```python
from build123d import *

# Parameters (mm, degrees)
BOSS_EXTRUDE1_DEPTH = 80
CUT_EXTRUDE1_REACH  = 152.333
CUT_EXTRUDE2_REACH  = 152.333
CUT_EXTRUDE3_REACH  = 152.333
SKETCH4_R           = 3
CUT_EXTRUDE4_REACH  = 152.333
SKETCH5_R           = 2.5
SKETCH5_R_2         = 3


with BuildPart() as part:
    # Sketch1 → Boss-Extrude1 (new body)
    with BuildSketch(Plane(origin=(0, 0, 0), x_dir=(1, 0, 0), z_dir=(0, 1, 0))):
        Polygon((0, 0), (90, 0), (90, 10), (10, 10), (10, 90), (0, 90), align=None)
    extrude(amount=BOSS_EXTRUDE1_DEPTH)

    # Sketch2 → Cut-Extrude1 (cut, up to next)
    with BuildSketch(Plane.XY, mode=Mode.PRIVATE) as cut_extrude1_sk1:
        Polygon((45, 80), (90, 40), (90, 80), align=None)
    cut_extrude1_tool1 = extrude(cut_extrude1_sk1.sketch, amount=-CUT_EXTRUDE1_REACH, mode=Mode.PRIVATE) & part.part
    add(cut_extrude1_tool1.solids().sort_by_distance((75, 66.666667, 0))[0], mode=Mode.SUBTRACT)

    # Sketch3 → Cut-Extrude2 (cut, up to next)
    with BuildSketch(Plane.ZY, mode=Mode.PRIVATE) as cut_extrude2_sk1:
        Polygon((-45, 80), (-90, 40), (-90, 80), align=None)
    cut_extrude2_tool1 = extrude(cut_extrude2_sk1.sketch, amount=-CUT_EXTRUDE2_REACH, mode=Mode.PRIVATE) & part.part
    add(cut_extrude2_tool1.solids().sort_by_distance((0, 66.666667, -75))[0], mode=Mode.SUBTRACT)

    # Sketch4 → Cut-Extrude3 (cut, up to next)
    with BuildSketch(Plane.XY, mode=Mode.PRIVATE) as cut_extrude3_sk1:
        with Locations((20, 70)):
            Circle(SKETCH4_R)
    cut_extrude3_tool1 = extrude(cut_extrude3_sk1.sketch, amount=-CUT_EXTRUDE3_REACH, mode=Mode.PRIVATE) & part.part
    # Sketch4 → Cut-Extrude3 (cut, up to next)
    with BuildSketch(Plane.XY, mode=Mode.PRIVATE) as cut_extrude3_sk2:
        with Locations((40, 70)):
            Circle(SKETCH4_R)
    cut_extrude3_tool2 = extrude(cut_extrude3_sk2.sketch, amount=-CUT_EXTRUDE3_REACH, mode=Mode.PRIVATE) & part.part
    # Sketch4 → Cut-Extrude3 (cut, up to next)
    with BuildSketch(Plane.XY, mode=Mode.PRIVATE) as cut_extrude3_sk3:
        with Locations((40, 50)):
            Circle(SKETCH4_R)
    cut_extrude3_tool3 = extrude(cut_extrude3_sk3.sketch, amount=-CUT_EXTRUDE3_REACH, mode=Mode.PRIVATE) & part.part
    # Sketch4 → Cut-Extrude3 (cut, up to next)
    with BuildSketch(Plane.XY, mode=Mode.PRIVATE) as cut_extrude3_sk4:
        with Locations((20, 30)):
            Circle(SKETCH4_R)
    cut_extrude3_tool4 = extrude(cut_extrude3_sk4.sketch, amount=-CUT_EXTRUDE3_REACH, mode=Mode.PRIVATE) & part.part
    # Sketch4 → Cut-Extrude3 (cut, up to next)
    with BuildSketch(Plane.XY, mode=Mode.PRIVATE) as cut_extrude3_sk5:
        with Locations((40, 10)):
            Circle(SKETCH4_R)
    cut_extrude3_tool5 = extrude(cut_extrude3_sk5.sketch, amount=-CUT_EXTRUDE3_REACH, mode=Mode.PRIVATE) & part.part
    # Sketch4 → Cut-Extrude3 (cut, up to next)
    with BuildSketch(Plane.XY, mode=Mode.PRIVATE) as cut_extrude3_sk6:
        with Locations((20, 50)):
            Circle(SKETCH4_R)
    cut_extrude3_tool6 = extrude(cut_extrude3_sk6.sketch, amount=-CUT_EXTRUDE3_REACH, mode=Mode.PRIVATE) & part.part
    # Sketch4 → Cut-Extrude3 (cut, up to next)
    with BuildSketch(Plane.XY, mode=Mode.PRIVATE) as cut_extrude3_sk7:
        with Locations((40, 30)):
            Circle(SKETCH4_R)
    cut_extrude3_tool7 = extrude(cut_extrude3_sk7.sketch, amount=-CUT_EXTRUDE3_REACH, mode=Mode.PRIVATE) & part.part
    # Sketch4 → Cut-Extrude3 (cut, up to next)
    with BuildSketch(Plane.XY, mode=Mode.PRIVATE) as cut_extrude3_sk8:
        with Locations((20, 10)):
            Circle(SKETCH4_R)
    cut_extrude3_tool8 = extrude(cut_extrude3_sk8.sketch, amount=-CUT_EXTRUDE3_REACH, mode=Mode.PRIVATE) & part.part
    # Sketch4 → Cut-Extrude3 (cut, up to next)
    with BuildSketch(Plane.XY, mode=Mode.PRIVATE) as cut_extrude3_sk9:
        with Locations((60, 30)):
            Circle(SKETCH4_R)
    cut_extrude3_tool9 = extrude(cut_extrude3_sk9.sketch, amount=-CUT_EXTRUDE3_REACH, mode=Mode.PRIVATE) & part.part
    # Sketch4 → Cut-Extrude3 (cut, up to next)
    with BuildSketch(Plane.XY, mode=Mode.PRIVATE) as cut_extrude3_sk10:
        with Locations((80, 10)):
            Circle(SKETCH4_R)
    cut_extrude3_tool10 = extrude(cut_extrude3_sk10.sketch, amount=-CUT_EXTRUDE3_REACH, mode=Mode.PRIVATE) & part.part
    # Sketch4 → Cut-Extrude3 (cut, up to next)
    with BuildSketch(Plane.XY, mode=Mode.PRIVATE) as cut_extrude3_sk11:
        with Locations((80, 30)):
            Circle(SKETCH4_R)
    cut_extrude3_tool11 = extrude(cut_extrude3_sk11.sketch, amount=-CUT_EXTRUDE3_REACH, mode=Mode.PRIVATE) & part.part
    # Sketch4 → Cut-Extrude3 (cut, up to next)
    with BuildSketch(Plane.XY, mode=Mode.PRIVATE) as cut_extrude3_sk12:
        with Locations((60, 10)):
            Circle(SKETCH4_R)
    cut_extrude3_tool12 = extrude(cut_extrude3_sk12.sketch, amount=-CUT_EXTRUDE3_REACH, mode=Mode.PRIVATE) & part.part
    add(cut_extrude3_tool1.solids().sort_by_distance((20, 70, 0))[0], mode=Mode.SUBTRACT)
    add(cut_extrude3_tool2.solids().sort_by_distance((40, 70, 0))[0], mode=Mode.SUBTRACT)
    add(cut_extrude3_tool3.solids().sort_by_distance((40, 50, 0))[0], mode=Mode.SUBTRACT)
    add(cut_extrude3_tool4.solids().sort_by_distance((20, 30, 0))[0], mode=Mode.SUBTRACT)
    add(cut_extrude3_tool5.solids().sort_by_distance((40, 10, 0))[0], mode=Mode.SUBTRACT)
    add(cut_extrude3_tool6.solids().sort_by_distance((20, 50, 0))[0], mode=Mode.SUBTRACT)
    add(cut_extrude3_tool7.solids().sort_by_distance((40, 30, 0))[0], mode=Mode.SUBTRACT)
    add(cut_extrude3_tool8.solids().sort_by_distance((20, 10, 0))[0], mode=Mode.SUBTRACT)
    add(cut_extrude3_tool9.solids().sort_by_distance((60, 30, 0))[0], mode=Mode.SUBTRACT)
    add(cut_extrude3_tool10.solids().sort_by_distance((80, 10, 0))[0], mode=Mode.SUBTRACT)
    add(cut_extrude3_tool11.solids().sort_by_distance((80, 30, 0))[0], mode=Mode.SUBTRACT)
    add(cut_extrude3_tool12.solids().sort_by_distance((60, 10, 0))[0], mode=Mode.SUBTRACT)

    # Sketch5 → Cut-Extrude4 (cut, up to next)
    with BuildSketch(Plane.ZY, mode=Mode.PRIVATE) as cut_extrude4_sk1:
        with Locations((-20, 30)):
            Circle(SKETCH5_R)
    cut_extrude4_tool1 = extrude(cut_extrude4_sk1.sketch, amount=-CUT_EXTRUDE4_REACH, mode=Mode.PRIVATE) & part.part
    # Sketch5 → Cut-Extrude4 (cut, up to next)
    with BuildSketch(Plane.ZY, mode=Mode.PRIVATE) as cut_extrude4_sk2:
        with Locations((-40, 30)):
            Circle(SKETCH5_R)
    cut_extrude4_tool2 = extrude(cut_extrude4_sk2.sketch, amount=-CUT_EXTRUDE4_REACH, mode=Mode.PRIVATE) & part.part
    # Sketch5 → Cut-Extrude4 (cut, up to next)
    with BuildSketch(Plane.ZY, mode=Mode.PRIVATE) as cut_extrude4_sk3:
        with Locations((-40, 10)):
            Circle(SKETCH5_R)
    cut_extrude4_tool3 = extrude(cut_extrude4_sk3.sketch, amount=-CUT_EXTRUDE4_REACH, mode=Mode.PRIVATE) & part.part
    # Sketch5 → Cut-Extrude4 (cut, up to next)
    with BuildSketch(Plane.ZY, mode=Mode.PRIVATE) as cut_extrude4_sk4:
        with Locations((-20, 10)):
            Circle(SKETCH5_R)
    cut_extrude4_tool4 = extrude(cut_extrude4_sk4.sketch, amount=-CUT_EXTRUDE4_REACH, mode=Mode.PRIVATE) & part.part
    # Sketch5 → Cut-Extrude4 (cut, up to next)
    with BuildSketch(Plane.ZY, mode=Mode.PRIVATE) as cut_extrude4_sk5:
        with Locations((-20, 70)):
            Circle(SKETCH5_R_2)
    cut_extrude4_tool5 = extrude(cut_extrude4_sk5.sketch, amount=-CUT_EXTRUDE4_REACH, mode=Mode.PRIVATE) & part.part
    # Sketch5 → Cut-Extrude4 (cut, up to next)
    with BuildSketch(Plane.ZY, mode=Mode.PRIVATE) as cut_extrude4_sk6:
        with Locations((-40, 70)):
            Circle(SKETCH5_R_2)
    cut_extrude4_tool6 = extrude(cut_extrude4_sk6.sketch, amount=-CUT_EXTRUDE4_REACH, mode=Mode.PRIVATE) & part.part
    # Sketch5 → Cut-Extrude4 (cut, up to next)
    with BuildSketch(Plane.ZY, mode=Mode.PRIVATE) as cut_extrude4_sk7:
        with Locations((-40, 50)):
            Circle(SKETCH5_R_2)
    cut_extrude4_tool7 = extrude(cut_extrude4_sk7.sketch, amount=-CUT_EXTRUDE4_REACH, mode=Mode.PRIVATE) & part.part
    # Sketch5 → Cut-Extrude4 (cut, up to next)
    with BuildSketch(Plane.ZY, mode=Mode.PRIVATE) as cut_extrude4_sk8:
        with Locations((-20, 50)):
            Circle(SKETCH5_R_2)
    cut_extrude4_tool8 = extrude(cut_extrude4_sk8.sketch, amount=-CUT_EXTRUDE4_REACH, mode=Mode.PRIVATE) & part.part
    # Sketch5 → Cut-Extrude4 (cut, up to next)
    with BuildSketch(Plane.ZY, mode=Mode.PRIVATE) as cut_extrude4_sk9:
        with Locations((-60, 30)):
            Circle(SKETCH5_R_2)
    cut_extrude4_tool9 = extrude(cut_extrude4_sk9.sketch, amount=-CUT_EXTRUDE4_REACH, mode=Mode.PRIVATE) & part.part
    # Sketch5 → Cut-Extrude4 (cut, up to next)
    with BuildSketch(Plane.ZY, mode=Mode.PRIVATE) as cut_extrude4_sk10:
        with Locations((-80, 30)):
            Circle(SKETCH5_R_2)
    cut_extrude4_tool10 = extrude(cut_extrude4_sk10.sketch, amount=-CUT_EXTRUDE4_REACH, mode=Mode.PRIVATE) & part.part
    # Sketch5 → Cut-Extrude4 (cut, up to next)
    with BuildSketch(Plane.ZY, mode=Mode.PRIVATE) as cut_extrude4_sk11:
        with Locations((-80, 10)):
            Circle(SKETCH5_R_2)
    cut_extrude4_tool11 = extrude(cut_extrude4_sk11.sketch, amount=-CUT_EXTRUDE4_REACH, mode=Mode.PRIVATE) & part.part
    # Sketch5 → Cut-Extrude4 (cut, up to next)
    with BuildSketch(Plane.ZY, mode=Mode.PRIVATE) as cut_extrude4_sk12:
        with Locations((-60, 10)):
            Circle(SKETCH5_R_2)
    cut_extrude4_tool12 = extrude(cut_extrude4_sk12.sketch, amount=-CUT_EXTRUDE4_REACH, mode=Mode.PRIVATE) & part.part
    add(cut_extrude4_tool1.solids().sort_by_distance((0, 30, -20))[0], mode=Mode.SUBTRACT)
    add(cut_extrude4_tool2.solids().sort_by_distance((0, 30, -40))[0], mode=Mode.SUBTRACT)
    add(cut_extrude4_tool3.solids().sort_by_distance((0, 10, -40))[0], mode=Mode.SUBTRACT)
    add(cut_extrude4_tool4.solids().sort_by_distance((0, 10, -20))[0], mode=Mode.SUBTRACT)
    add(cut_extrude4_tool5.solids().sort_by_distance((0, 70, -20))[0], mode=Mode.SUBTRACT)
    add(cut_extrude4_tool6.solids().sort_by_distance((0, 70, -40))[0], mode=Mode.SUBTRACT)
    add(cut_extrude4_tool7.solids().sort_by_distance((0, 50, -40))[0], mode=Mode.SUBTRACT)
    add(cut_extrude4_tool8.solids().sort_by_distance((0, 50, -20))[0], mode=Mode.SUBTRACT)
    add(cut_extrude4_tool9.solids().sort_by_distance((0, 30, -60))[0], mode=Mode.SUBTRACT)
    add(cut_extrude4_tool10.solids().sort_by_distance((0, 30, -80))[0], mode=Mode.SUBTRACT)
    add(cut_extrude4_tool11.solids().sort_by_distance((0, 10, -80))[0], mode=Mode.SUBTRACT)
    add(cut_extrude4_tool12.solids().sort_by_distance((0, 10, -60))[0], mode=Mode.SUBTRACT)


solid = part.part
```
Read the model definition and answer for the solid it produces. Units are mm, in the model's axes. A direction names the side the tool comes from. Coordinates: 2 decimals unless noted, no trailing zeros. Order: outer loops, then holes, each group sorted by start corner. A loop starts at its lowest first (then second) coordinate and runs counter-clockwise, first axis right, second up. Notation, with made-up numbers: (-14, 77) - (21, 77) arc R16 cw to (21, 91) - close; hole circle Ø5 at (13, 3). An arc over 180 degrees is marked (long way). Answer as a JSON object with one key per item and string values. Group by question number.
Item 1: Section C-C (x = 60) is taken. Give the vertices of the cut face in (y, z), plus the area to 3 significant figures.
Item 2: Section A-A (y = 70) is taken. Give the vertices of the cut face in (x, z), plus the area to 3 significant figures.
Item 3: Consider probe 1 along Y at (x, z) = (20, -8); probe 2 along Y at (x, z) = (2, -60); probe 3 along Y at (x, z) = (7, -62). Determine where each line is inside the solid, lowest interval first. Write a range as from..to.
Item 4: Flat-ended cylindrical pins translate along their axes: P1, Ø5, axis at y = 23, z = -30, coming from the -X side; P2, Ø24, axis at x = 65.5, y = 36, coming from the -Z side; P3, Ø6.5, axis at y = 10, z = -20, coming from the +X side. Find the tip coordinate at first contact, or state that the pin passes through.
Item 5: Section D-D (z = -60) is taken. Give the vertices of the cut face in (x, y).
Item 6: The mould has two halves that part along Z. Classify faces 1 (the face through (5, 53, -20)), 2 (the face through (57, 30, -5)), 3 (the face through (42, 39, -10)): +Z half, -Z half, draft (parallel to the pull), parting line (faces both ways), or undercut.
Item 7: Section B-B (z = -20) is taken. Give the vertices of the cut face in (x, y), plus the area to 3 significant figures.
Item 8: A tool of negligible diameter and unlimited length cuts with its end or side. For faces 4 (the face through (10, 39, -49)), 5 (the face through (19.35, 67.07, -4.93)), from which of +Z, -Z, +X, -X, +Y, -Y can it reach the whole face along a straight path? Write none if from no direction.
Results are:
{
 "1": {"outline": "(0, -10) - (7, -10) - (7, 0) - (0, 0) - close; (13, -10) - (27, -10) - (27, 0) - (13, 0) - close; (33, -10) - (66.67, -10) - (66.67, 0) - (33, 0) - close", "area": "547 mm^2"},
 "2": {"outline": "(0, -56.25) - (10, -56.25) - (10, -43) - (0, -43) - close; (0, -37) - (10, -37) - (10, -23) - (0, -23) - close; (0, -17) - (10, -17) - (10, -10) - (17, -10) - (17, 0) - (0, 0) - close; (23, -10) - (37, -10) - (37, 0) - (23, 0) - close; (43, -10) - (56.25, -10) - (56.25, 0) - (43, 0) - close", "area": "785 mm^2"},
 "3": {"probe 1": "y = 0..7, 13..27, 33..47, 53..67, 73..80", "probe 2": "y = 0..7, 13..27, 33..66.67", "probe 3": "y = 0..7.76, 12.24..27.76, 32.24..64.89"},
 "4": {"P1": "stops at x = 0", "P2": "stops at z = -10", "P3": "stops at x = 10"},
 "5": {"outline": "(0, 0) - (10, 0) - (10, 7) - (0, 7) - close; (0, 13) - (10, 13) - (10, 27) - (0, 27) - close; (0, 33) - (10, 33) - (10, 66.67) - (0, 66.67) - close"},
 "6": {"face 1": "undercut", "face 2": "draft", "face 3": "-Z half"},
 "7": {"outline": "(0, 0) - (10, 0) - (10, 7.5) - (0, 7.5) - close; (0, 12.5) - (10, 12.5) - (10, 27.5) - (0, 27.5) - close; (0, 32.5) - (10, 32.5) - (10, 47) - (0, 47) - close; (0, 53) - (10, 53) - (10, 67) - (0, 67) - close; (0, 73) - (10, 73) - (10, 80) - (0, 80) - close", "area": "580 mm^2"},
 "8": {"face 4": "-Z, +X, +Y, -Y", "face 5": "+Z, -Z"}
}
